from build123d import *

# Parameters (mm, degrees)
SKETCH1_W                      = 50.8
SKETCH1_H                      = 90
MAIN_EXTRUDE_DEPTH             = 30
SKETCH2_R                      = 12.75
MOTOR_SLOT_CUT_DEPTH           = 64
SKETCH3_W                      = 8.3
SKETCH3_H                      = 25
FILLAMENT_THROUGHWAY_CUT_DEPTH = 51.8
SKETCH4_R                      = 3.175
BOTTOM_AXLE_CUT_DEPTH          = 91
SKETCH6_W                      = 50.8
SKETCH6_H                      = 4.35
SKETCH6_H_2                    = 5
TOP_FINS_EXTRUDE_DEPTH         = 18.15
TOP_AXLE_CUT_DEPTH             = 91
SKETCH8_W                      = 15
SKETCH8_H                      = 15
WIRE_HOLE_CUT_DEPTH            = 8
SKETCH9_W                      = 19.4
SKETCH9_H                      = 43.140250719
EASEOFACCESSCUT_DEPTH          = 20
SKETCH10_W                     = 25
SKETCH10_H                     = 27.637362277
BEARINGSIZECUT_DEPTH           = 5.5
SKETCH11_W                     = 10
SKETCH11_H                     = 25.030494578
RUBBER_BAND_CUT_DEPTH          = 51.8
SKETCH12_W                     = 50.8
SKETCH12_H                     = 5.009749281
BOSS_EXTRUDE1_DEPTH            = 12.41
SKETCH13_W                     = 12
SKETCH13_H                     = 4.924328521
BOSS_EXTRUDE2_DEPTH            = 43.140251
SKETCH15_R                     = 3.175
CUT_EXTRUDE1_DEPTH             = 12.41


with BuildPart() as part:
    # Sketch1 → Main Extrude (new body)
    with BuildSketch(Plane(origin=(0, 0, 0), x_dir=(1, 0, 0), z_dir=(0, 1, 0))):
        Rectangle(SKETCH1_W, SKETCH1_H)
    extrude(amount=MAIN_EXTRUDE_DEPTH)

    # Sketch2 → Motor Slot Cut (cut)
    with BuildSketch(Plane(origin=(0, 0, -45), x_dir=(-1, 0, 0), z_dir=(0, 0, -1))):
        with Locations((0, 15)):
            Circle(SKETCH2_R)
    extrude(amount=-MOTOR_SLOT_CUT_DEPTH, mode=Mode.SUBTRACT)

    # Sketch3 → Fillament Throughway cut (cut, through all)
    with BuildSketch(Plane(origin=(25.4, 0, 0), x_dir=(0, 0, -1), z_dir=(1, 0, 0))):
        with Locations((-36.5, 17.5)):
            Rectangle(SKETCH3_W, SKETCH3_H)
    extrude(amount=-FILLAMENT_THROUGHWAY_CUT_DEPTH, mode=Mode.SUBTRACT)

    # Sketch4 → Bottom Axle Cut (cut, through all)
    with BuildSketch(Plane.XY.offset(45)):
        with Locations((0, 15)):
            Circle(SKETCH4_R)
    extrude(amount=-BOTTOM_AXLE_CUT_DEPTH, mode=Mode.SUBTRACT)

    # Sketch6 → Top Fins Extrude (add)
    with BuildSketch(Plane(origin=(0, 30, 0), x_dir=(1, 0, 0), z_dir=(0, 1, 0))):
        with Locations((0, -42.825)):
            Rectangle(SKETCH6_W, SKETCH6_H)
        with Locations((0, -29.85)):
            Rectangle(SKETCH6_W, SKETCH6_H_2)
    extrude(amount=TOP_FINS_EXTRUDE_DEPTH)

    # Sketch7 → Top Axle Cut (cut, through all)
    with BuildSketch(Plane.XY.offset(45)):
        with BuildLine():
            Line((2.54, 43.275), (2.54, 33.275))
            ThreePointArc((2.54, 33.275), (0, 30.735), (-2.54, 33.275))
            Line((-2.54, 33.275), (-2.54, 43.275))
            ThreePointArc((-2.54, 43.275), (0, 45.815), (2.54, 43.275))
        make_face()
    extrude(amount=-TOP_AXLE_CUT_DEPTH, mode=Mode.SUBTRACT)

    # Sketch8 → Wire Hole Cut (cut)
    with BuildSketch(Plane(origin=(0, 30, 0), x_dir=(1, 0, 0), z_dir=(0, 1, 0))):
        with Locations((0, 37.5)):
            Rectangle(SKETCH8_W, SKETCH8_H)
    extrude(amount=-WIRE_HOLE_CUT_DEPTH, mode=Mode.SUBTRACT)

    # Sketch9 → EaseOfAccessCut (cut)
    with BuildSketch(Plane.XY.offset(45)):
        with Locations((-15.7, 26.579874641)):
            Rectangle(SKETCH9_W, SKETCH9_H)
        with Locations((15.7, 26.579874641)):
            Rectangle(SKETCH9_W, SKETCH9_H)
    extrude(amount=-EASEOFACCESSCUT_DEPTH, mode=Mode.SUBTRACT)

    # Sketch10 → BearingSizeCut (cut, symmetric)
    with BuildSketch(Plane.XY.offset(36.5)):
        with Locations((0, 38.093681139)):
            Rectangle(SKETCH10_W, SKETCH10_H)
    extrude(amount=BEARINGSIZECUT_DEPTH, both=True, mode=Mode.SUBTRACT)

    # Sketch11 → Rubber Band Cut (cut, through all)
    with BuildSketch(Plane(origin=(25.4, 0, 0), x_dir=(0, 0, -1), z_dir=(1, 0, 0))):
        with Locations((-22.35, 17.484752711)):
            Rectangle(SKETCH11_W, SKETCH11_H)
    extrude(amount=-RUBBER_BAND_CUT_DEPTH, mode=Mode.SUBTRACT)

    # Sketch12 → Boss-Extrude1 (add)
    with BuildSketch(Plane.XY.offset(45)):
        with Locations((0, 2.504874641)):
            Rectangle(SKETCH12_W, SKETCH12_H)
    extrude(amount=BOSS_EXTRUDE1_DEPTH)

    # Sketch13 → Boss-Extrude2 (add)
    with BuildSketch(Plane(origin=(0, 5.009749281, 0), x_dir=(1, 0, 0), z_dir=(0, 1, 0))):
        with Locations((0, -54.94783574)):
            Rectangle(SKETCH13_W, SKETCH13_H)
    extrude(amount=BOSS_EXTRUDE2_DEPTH)

    # Sketch15 → Cut-Extrude1 (cut)
    with BuildSketch(Plane(origin=(0, 0, 52.485671479), x_dir=(-1, 0, 0), z_dir=(0, 0, -1))):
        with Locations((0, 15)):
            Circle(SKETCH15_R)
        with BuildLine():
            Line((-2.54, 33.28), (-2.54, 43.28))
            ThreePointArc((-2.54, 43.28), (0, 45.82), (2.54, 43.28))
            Line((2.54, 43.28), (2.54, 33.28))
            ThreePointArc((2.54, 33.28), (0, 30.74), (-2.54, 33.28))
        make_face()
    extrude(amount=-CUT_EXTRUDE1_DEPTH, mode=Mode.SUBTRACT)


solid = part.part
Can you work these out from the model? Positions are in its coordinate system, mm. A direction names the side the tool comes from. Give positions to 0.01 mm unless a question says otherwise; leave off trailing zeros. Loops run counter-clockwise (first coordinate to the right, second up) from the corner with the lowest first, then second, coordinate; pieces in that order, holes last. Notation, with made-up numbers: (68.25, 30) -> (110.25, 30) arc R13 ccw to (110.25, 42) -> close; hole circle Ø8 at (-8, -40). An arc over 180 degrees is marked (long way). Return JSON: item names as keys, results as strings.
Q1. We'd pull the mould along X, two halves only. Please class faces 5 (the face through (0, 4.97, 22)), 6 (the face through (-6, 26, 43)), 7 (the face through (-0.06, 30.74, 54.91)): released by +X, released by -X, zero draft, split by the parting line, or undercut.
Checks:
{"face 5": "zero draft", "face 6": "released by -X", "face 7": "undercut"}
Q2. I want a section at C-C, the plane z = -4. List the corners of the cut face in (x, y) for me.
Checks:
{"outline": "(-25.4, 0) -> (25.4, 0) -> (25.4, 30) -> (-25.4, 30) -> close; hole circle Ø25.5 at (0, 15)"}
Q3. On a 3-axis mill with a long thin cutter (end or side, diameter ignored), from which of +Z, -Z, +X, -X, +Y, -Y can I reach the whole of each face in a straight line? I mean faces 1 (the face through (0, 48.15, 55)), 2 (the face through (-7.5, 28, -37)), 3 (the face through (0.056, 30.736, 29.201)), 4 (the face through (0, 26, 45)). Say none if no direction works.
Checks:
{"face 1": "+Z, -Z, +X, -X, +Y", "face 2": "-Z, +Y", "face 3": "+Z, -Z", "face 4": "+X, -X, +Y"}
Q4. I want a section at A-A, the plane y = 38. List the corners of the cut face in (x, z) for me.
Checks:
{"outline": "(-6, 27.35) -> (-2.54, 27.35) -> (-2.54, 31) -> (-6, 31) -> close; (-6, 42) -> (-2.54, 42) -> (-2.54, 45) -> (-6, 45) -> close; (-6, 52.49) -> (-2.54, 52.49) -> (-2.54, 57.41) -> (-6, 57.41) -> close; (2.54, 27.35) -> (6, 27.35) -> (6, 31) -> (2.54, 31) -> close; (2.54, 42) -> (6, 42) -> (6, 45) -> (2.54, 45) -> close; (2.54, 52.49) -> (6, 52.49) -> (6, 57.41) -> (2.54, 57.41) -> close"}
Q5. I need wall thicknesses on probe 1 along Z at (x, y) = (1.5, 46); probe 2 along Z at (x, y) = (-4.5, 18); probe 3 along Y at (x, z) = (0, -20). Which ranges of each line are inside material? Lowest first, please.
Checks:
{"probe 1": "z = 27.35 to 31, 42 to 45, 52.49 to 57.41", "probe 2": "z = 27.35 to 32.35, 40.65 to 45, 52.49 to 57.41", "probe 3": "y = 0 to 2.25, 27.75 to 30"}
Q6. For pin 1 Ø1.4 at (x, y) = (-2.5, 4) entering from -Z; pin 2 Ø6 at (x, y) = (3.5, 17) entering from -Z; pin 3 Ø2.5 at (x, y) = (2.5, 28) entering from -Z, each with a flat end and sliding along its axis, tell me the tip position at first contact or that it passes through.
Checks:
{"pin 1": "stops at z = 19", "pin 2": "stops at z = 27.35", "pin 3": "stops at z = -30"}
